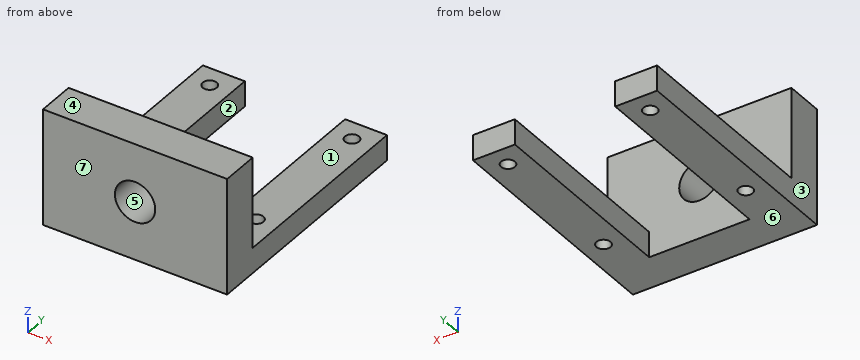
Autodesk Inventor part; units mm, degrees
ref_plane "YZ Plane" through (0, 0, 0) normal (1, 0, 0) x (0, 1, 0)
ref_plane "XZ Plane" through (0, 0, 0) normal (0, 1, 0) x (-1, 0, 0)
ref_plane "XY Plane" through (0, 0, 0) normal (0, 0, 1) x (1, 0, 0)
sketch "Sketch1" plane through (0, 0, 0) normal (0, 1, 0) x (-1, 0, 0)
  line L0 (0, 0) -> (29, 0)
  line L1 (29, 0) -> (29, 18.3)
  line L2 (29, 18.3) -> (0, 18.3)
  line L3 (0, 18.3) -> (0, 0)
  dimension "d0" = 29
  dimension "d1" = 18.3
extrude "Extrusion1" add sketch "Sketch1" along normal blind 6
sketch "Sketch2" plane through (0, 6, 0) normal (0, 1, 0) x (1, 0, 0)
  line L0 (0, 0) -> (-29, 0)
  line L1 (0, 0) -> (-6.6, 0)
  line L2 (-6.6, 0) -> (-6.6, -4)
  line L3 (-6.6, -4) -> (0, -4)
  line L4 (0, -4) -> (0, 0)
  dimension "d4" = 6.6
  dimension "d5" = 4
extrude "Extrusion2" add sketch "Sketch2" along normal blind 31.5
sketch "Sketch3" plane through (0, 6, 0) normal (0, 1, 0) x (1, 0, 0)
  line L0 (-6.6, 0) -> (-29, 0)
  line L1 (-29, 0) -> (-22.4, 0)
  line L2 (-22.4, 0) -> (-22.4, -4)
  line L3 (-22.4, -4) -> (-29, -4)
  line L4 (-29, -4) -> (-29, 0)
  point P0 (0, 0)
  dimension "d8" = 6.6
  dimension "d9" = 4
extrude "Extrusion3" add sketch "Sketch3" along normal blind 31.5
sketch "Sketch4" plane through (-6.6, 6, 4) normal (0, 0, 1) x (1, 0, 0)
  line L0 (-22.4, 0) -> (6.6, 0)
  point P0 (6.6, -6)
  point P1 (3.3, 5.8)
  point P2 (3.3, 5.8)
  point P3 (3.3, 28.2)
  point P4 (-19.1, 5.8)
  point P5 (-19.1, 28.2)
  dimension "d14" = 5.8
  dimension "d15" = 22.4
  dimension "d16" = 22.4
  dimension "d17" = 22.4
  dimension "d18" = 5.8
hole "Hole1" at (-3.3, 11.8, 4) at (-3.3, 34.2, 4) at (-25.7, 11.8, 4) at (-25.7, 34.2, 4) direction (0, 0, -1) diameter 2.2 end through all
sketch "Sketch5" plane through (-29, 0, 18.3) normal (0, 0, 1) x (1, 0, 0)
  point P0 (29, 0)
sketch "Sketch6" plane through (0, 0, 0) normal (0, -1, 0) x (1, 0, 0)
  line L0 (-29, 18.3) -> (0, 18.3)
  point P0 (0, 0)
  point P1 (-14.5, 9.15)
  dimension "d26" = 9.15
hole "Hole2" at (-14.5, 0, 9.15) direction (0, 1, 0) diameter 6.35 end through all
properties part number "adapter"
Geometry: final body of the model. Coordinates: model frame, mm. Face numbers are marked on the shaded views. A direction names the side the tool comes from. Give positions to 0.01 mm unless a question says otherwise; leave off trailing zeros. Order: outer loops, then holes, each group sorted by start corner. A loop starts at its lowest first (then second) coordinate and runs counter-clockwise, first axis right, second up. Notation, with made-up numbers: (12.25, 61.25) -> (39.25, 61.25) arc R19 ccw to (39.25, 87.25) -> close; hole circle Ø4 at (38, -29). An arc over 180 degrees is marked (long way). Write each question's results on one line, items separated by ' | '.
1) Cut plane C-C (z = 9.15). Output: boundary loops of the cut face in (x, y) (3 decimals).
Geometry says:
outline: (-29, 0) -> (-17.675, 0) -> (-17.675, 6) -> (-29, 6) -> close; (-11.325, 0) -> (0, 0) -> (0, 6) -> (-11.325, 6) -> close
2) Cut plane B-B (y = 27.5). Output: boundary loops of the cut face in (x, z), and give its area (3 significant figures).
Geometry says:
outline: (-29, 0) -> (-22.4, 0) -> (-22.4, 4) -> (-29, 4) -> close; (-6.6, 0) -> (0, 0) -> (0, 4) -> (-6.6, 4) -> close | area: 52.8 mm²
3) Cut plane A-A (x = -25.7). Output: boundary loops of the cut face in (y, z), and give its area (3 significant figures).
Geometry says:
outline: (0, 0) -> (10.7, 0) -> (10.7, 4) -> (6, 4) -> (6, 18.3) -> (0, 18.3) -> close; (12.9, 0) -> (33.1, 0) -> (33.1, 4) -> (12.9, 4) -> close; (35.3, 0) -> (37.5, 0) -> (37.5, 4) -> (35.3, 4) -> close | area: 218 mm²
4) Line query: line 1 along X through (y, z) = (34.2, 1.4); line 2 along Y through (x, z) = (-25.7, 2.9); line 3 along X through (y, z) = (4.35, 9.15) (3 decimals). Output: solid intervals per line, ascending.
Geometry says:
line 1: x = -29 to -26.8, -24.6 to -22.4, -6.6 to -4.4, -2.2 to 0 | line 2: y = 0 to 10.7, 12.9 to 33.1, 35.3 to 37.5 | line 3: x = -29 to -17.675, -11.325 to 0
5) Draft query along Z for the marked faces 4, 5, 6 and 7. Return one class per face: released by +Z, released by -Z, zero draft, split by the parting line, or undercut.
Geometry says:
face 4: released by +Z | face 5: undercut | face 6: released by -Z | face 7: zero draft
6) First-contact query: pin 1 Ø1 at (x, z) = (-20, 14.5) entering from +Y; pin 2 Ø5.5 at (x, z) = (-14.5, 9.15) entering from -Y; pin 3 Ø3.5 at (x, y) = (-3.5, 17) entering from +Z. Flat tips, straight axial feed; report the tip coordinate or a pass-through.
Geometry says:
pin 1: stops at y = 6 | pin 2: passes through | pin 3: stops at z = 4
7) Cut plane D-D (y = 5.5). Output: boundary loops of the cut face in (x, z) (3 decimals), and give its area (3 significant figures).
Geometry says:
outline: (-29, 0) -> (0, 0) -> (0, 18.3) -> (-29, 18.3) -> close; hole circle Ø6.35 at (-14.5, 9.15) | area: 499 mm²
8) Set-up query: the marked faces 1, 2 and 3. Return all of +Z, -Z, +X, -X, +Y, -Y with unobstructed straight access to the full face (end or side cutting, diameter ignored); none if empty.
Geometry says:
face 1: +Z, +X, -X, +Y | face 2: +Z, -Z, +Y | face 3: +Z, -Z, -X, +Y, -Y
